Geometry check sheet. Reference: drawing and pictorial views, mm from the part's lowest x, y, z. Give positions to 0.01 mm unless a question says otherwise; leave off trailing zeros. Write each loop counter-clockwise with the first axis right and the second up, starting at its lowest first coordinate (ties: lowest second). Pieces come first, ordered by that corner, then holes. Notation, with made-up numbers: (38, 89) -> (62, 89) arc R23 ccw to (62, 97) -> close; hole circle Ø2 at (70.25, 1.5). An arc over 180 degrees is marked (long way). Use a Markdown table: item, result. Add a question column.
1. Cross-section at B-B (z = 11.43). Enter the section's corners in (x, y), then the cut area to 3 significant figures.
2. Scan lines: probe 1 along Z at (x, y) = (54.57, 5.5); probe 2 along Z at (x, y) = (31, 4); probe 3 along Z at (x, y) = (87.5, 3.75). Record each from-to range of solid material in increasing order. Write a range as [from, to].
3. Gauge pin test, flat end, axial feed: P1, Ø12, axis at x = 31, z = 35, coming from the +Y side. Record the tip position at first contact, or that the pin passes through.
4. Cross-section at A-A (x = 54.57). Enter the section's corners in (y, z).
5. Release check for a two-part mould opening along Z. For the marked faces 1, 2, 3 and 4 record: released by +Z, released by -Z, zero draft, split by the parting line, or undercut.
6. Cross-section at D-D (x = 31). Enter the section's corners in (y, z), then the cut area to 3 significant figures.
7. Cross-section at C-C (y = 2.5). Count the separate pieces of the cut face and the enclosed holes in it, then the cut area to 3 significant figures.
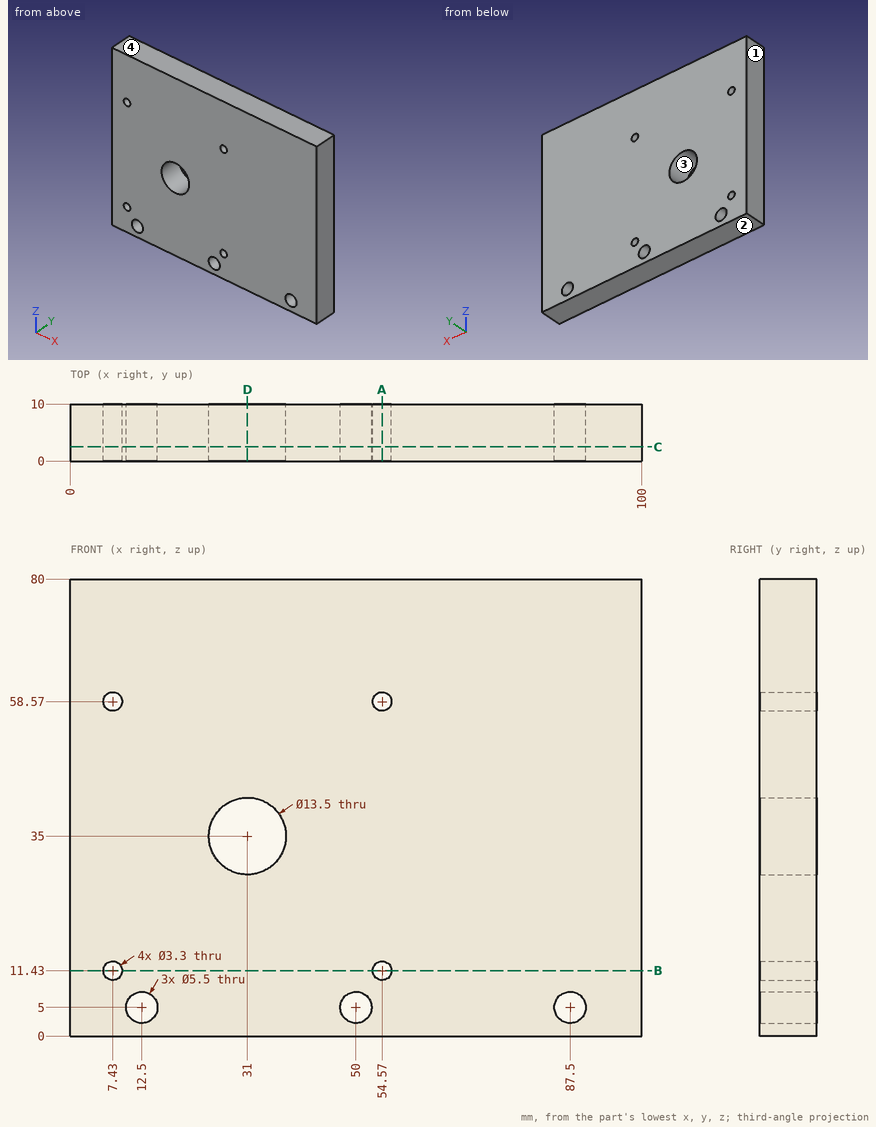
Worked answers:
| question | item | result |
|---|---|---|
| 1 | outline | (0, 0) -> (5.78, 0) -> (5.78, 10) -> (0, 10) -> close; (9.08, 0) -> (52.92, 0) -> (52.92, 10) -> (9.08, 10) -> close; (56.22, 0) -> (100, 0) -> (100, 10) -> (56.22, 10) -> close |
| 1 | area | 934 mm² |
| 2 | probe 1 | z = [0, 9.78], [13.08, 56.92], [60.22, 80] |
| 2 | probe 2 | z = [0, 28.25], [41.75, 80] |
| 2 | probe 3 | z = [0, 2.25], [7.75, 80] |
| 3 | P1 | passes through |
| 4 | outline | (0, 0) -> (10, 0) -> (10, 9.78) -> (0, 9.78) -> close; (0, 13.08) -> (10, 13.08) -> (10, 56.92) -> (0, 56.92) -> close; (0, 60.22) -> (10, 60.22) -> (10, 80) -> (0, 80) -> close |
| 5 | face 1 | zero draft |
| 5 | face 2 | released by -Z |
| 5 | face 3 | undercut |
| 5 | face 4 | released by +Z |
| 6 | outline | (0, 0) -> (10, 0) -> (10, 28.25) -> (0, 28.25) -> close; (0, 41.75) -> (10, 41.75) -> (10, 80) -> (0, 80) -> close |
| 6 | area | 665 mm² |
| 7 | separate pieces | 1 |
| 7 | enclosed holes | 8 |
| 7 | area | 7,750 mm² |
